For this review, take the finished solid that the model builds, in its own axes (mm). Give positions to 0.01 mm unless a question says otherwise; leave off trailing zeros. Loops run counter-clockwise (first coordinate to the right, second up) from the corner with the lowest first, then second, coordinate; pieces in that order, holes last. Notation, with made-up numbers: M 60.25,-25.5 L 86.25,-25.5 A18 cw 86.25,1.5 Z; hole C -12,-34 d7. An arc over 180 degrees is marked long. Use CSV: the item, a comma, the result in double quotes. Start each with the question number.
1. To check wall thickness, follow line 1 (Y direction, x = 0, z = 1.45); line 2 (X direction, y = -18.5, z = 1.3); line 3 (Y direction, x = 0, z = 1.05). State the ranges of each line that lie inside material, in increasing order. Write a range as [from, to].
2. Take a section at C-C, the plane z = -0.45. Write out the cut boundary in (x, y), and give its area (3 significant figures).
3. Insertion check: P1, Ø1, axis at y = -91.5, z = -0.5, coming from the -X side; P2, Ø1.5, axis at x = -63, z = 1, coming from the -Y side; P3, Ø8, axis at x = 0, y = 0, coming from the -Z side; P4, Ø1.5, axis at x = -28, y = 43, coming from the +Z side. Each pin has a flat end and moves straight along its axis. Give the tip position at first contact, or say it passes through.
4. Take a section at A-A, the plane x = 0. Write out the cut boundary in (y, z), and give its area (3 significant figures).
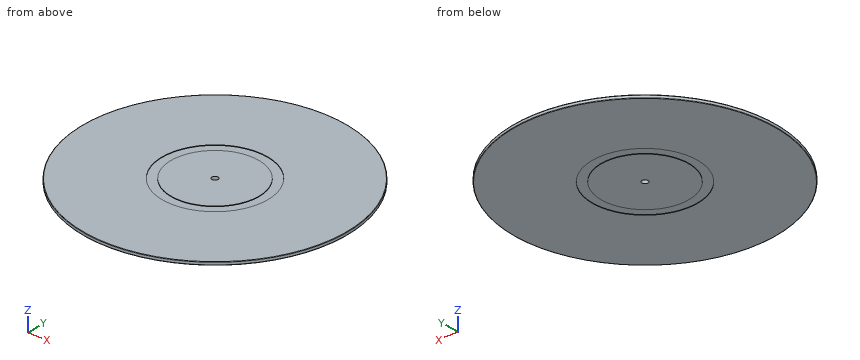
from build123d import *

# Parameters (mm, degrees)
SKETCH_R      = 150
SKETCH_R_2    = 3.5
PAD_DEPTH     = 1.75
FILLET_R      = 0.5
SKETCH001_R   = 60
SKETCH001_R_2 = 50
POCKET_DEPTH  = 0.5


with BuildPart() as part:
    # Sketch → Pad (new body, symmetric)
    with BuildSketch(Plane.XY):
        Circle(SKETCH_R)
        Circle(SKETCH_R_2, mode=Mode.SUBTRACT)
    extrude(amount=PAD_DEPTH, both=True)

    # Fillet
    fillet_edges = [part.edges().sort_by_distance(p)[0] for p in [
        (150, 0, 0),
        (-150, 0, -1.75),
        (-150, 0, 1.75),
    ]]
    fillet(fillet_edges, radius=FILLET_R)

    # Sketch001 → Pocket (cut)
    with BuildSketch(Plane.XY.offset(1.75)):
        Circle(SKETCH001_R)
        Circle(SKETCH001_R_2, mode=Mode.SUBTRACT)
    pocket = extrude(amount=-POCKET_DEPTH, mode=Mode.SUBTRACT)

    # Mirrored: Pocket across XY
    add(pocket.mirror(Plane.XY), mode=Mode.SUBTRACT)


solid = part.part
Result set:
1,line 1,"[-149.96, -60], [-50, -3.5], [3.5, 50], [60, 149.96]"
1,line 2,"[-148.85, -57.08], [-46.45, 46.45], [57.08, 148.85]"
1,line 3,"[-150, -3.5], [3.5, 150]"
2,outline,"C 0,0 d300; hole C 0,0 d7"
2,area,"70,600 mm2"
3,P1,"x = -119.24"
3,P2,"y = -136.47"
3,P3,"z = -1.75"
3,P4,"z = 1.25"
4,outline,"M -150,-1.25 A0.5 ccw -149.5,-1.75 L -60,-1.75 L -60,-1.25 L -50,-1.25 L -50,-1.75 L -3.5,-1.75 L -3.5,1.75 L -50,1.75 L -50,1.25 L -60,1.25 L -60,1.75 L -149.5,1.75 A0.5 ccw -150,1.25 Z; M 3.5,-1.75 L 50,-1.75 L 50,-1.25 L 60,-1.25 L 60,-1.75 L 149.5,-1.75 A0.5 ccw 150,-1.25 L 150,1.25 A0.5 ccw 149.5,1.75 L 60,1.75 L 60,1.25 L 50,1.25 L 50,1.75 L 3.5,1.75 Z"
4,area,"1,010 mm2"
